Geometry check sheet. Reference: the model listing, model coordinates, mm. A direction names the side the tool comes from. Give positions to 0.01 mm unless a question says otherwise; leave off trailing zeros. Order: outer loops, then holes, each group sorted by start corner. A loop starts at its lowest first (then second) coordinate and runs counter-clockwise, first axis right, second up. Notation, with made-up numbers: M 17.5,62.5 L 47.5,62.5 A17 ccw 47.5,79.5 Z; hole C 5,65 d2. An arc over 180 degrees is marked long. Answer as CSV lines item,"result".
from build123d import *

# Parameters (mm, degrees)
SKETCH1_R           = 6
BOSS_EXTRUDE1_DEPTH = 10
CUT_EXTRUDE1_REACH  = 34.013
CUT_EXTRUDE2_START  = -12.127591
CUT_EXTRUDE2_DEPTH  = 8.847142
BOSS_EXTRUDE7_DEPTH = 5
SKETCH3_R           = 1.25
CUT_EXTRUDE3_DEPTH  = 5
SKETCH3_2_R         = 1.25
CUT_EXTRUDE4_DEPTH  = 11.819305932


with BuildPart() as part:
    # Sketch1 → Boss-Extrude1 (new body)
    with BuildSketch(Plane(origin=(0, 0, 0), x_dir=(0, 0, -1), z_dir=(1, 0, 0))):
        with BuildLine():
            Line((-4.273163423, 7.920863233), (-4.273163423, 20.04845395))
            Line((-4.273163423, 20.04845395), (6, 20.04845395))
            Line((6, 20.04845395), (6, 17.649323049))
            Line((6, 17.649323049), (4.273163423, 17.649323049))
            Line((4.273163423, 17.649323049), (4.273163423, 16.76800454))
            Line((4.273163423, 16.76800454), (5.136581711, 16.76800454))
            Line((5.136581711, 16.76800454), (5.136581711, 15.879894787))
            Line((5.136581711, 15.879894787), (4.273163423, 15.879894787))
            Line((4.273163423, 15.879894787), (4.273163423, 14.998576279))
            Line((4.273163423, 14.998576279), (5.136581711, 14.998576279))
            Line((5.136581711, 14.998576279), (5.136581711, 14.110466526))
            Line((5.136581711, 14.110466526), (4.273163423, 14.110466526))
            Line((4.273163423, 14.110466526), (4.273163423, 13.229148017))
            Line((4.273163423, 13.229148017), (5.136581711, 13.229148017))
            Line((5.136581711, 13.229148017), (5.136581711, 12.341038265))
            Line((5.136581711, 12.341038265), (4.273163423, 12.341038265))
            Line((4.273163423, 12.341038265), (4.273163423, 11.459719756))
            Line((4.273163423, 11.459719756), (5.136581711, 11.459719756))
            Line((5.136581711, 11.459719756), (5.136581711, 10.571610003))
            Line((5.136581711, 10.571610003), (4.273163423, 10.571610003))
            Line((4.273163423, 10.571610003), (4.273163423, 9.690291495))
            Line((4.273163423, 9.690291495), (5.136581711, 9.690291495))
            Line((5.136581711, 9.690291495), (5.136581711, 8.802181742))
            Line((5.136581711, 8.802181742), (4.273163423, 8.802181742))
            Line((4.273163423, 8.802181742), (4.273163423, 7.920863233))
            ThreePointArc((4.273163423, 7.920863233), (0, -9), (-4.273163423, 7.920863233))
        make_face()
        Circle(SKETCH1_R, mode=Mode.SUBTRACT)
    extrude(amount=BOSS_EXTRUDE1_DEPTH)

    # Cut-Extrude1: up to this face of the body (flat: up to its plane)
    cut_extrude1_end = Plane(part.part.faces().sort_by_distance((5, 16.76800454, -4.704872567))[0])
    # Sketch2 → Cut-Extrude1 (cut, up to the picked face)
    with BuildSketch(Plane(origin=(0, 20.04845395, 0), x_dir=(1, 0, 0), z_dir=(0, 1, 0)), mode=Mode.PRIVATE) as cut_extrude1_sk1:
        Polygon((10, 6), (5, 6), (10, 1), align=None)
    cut_extrude1_tool1 = split(extrude(cut_extrude1_sk1.sketch, amount=-CUT_EXTRUDE1_REACH, mode=Mode.PRIVATE), bisect_by=cut_extrude1_end, keep=Keep.BOTH, mode=Mode.PRIVATE)
    # Sketch2 → Cut-Extrude1 (cut, up to the picked face)
    with BuildSketch(Plane(origin=(0, 20.04845395, 0), x_dir=(1, 0, 0), z_dir=(0, 1, 0)), mode=Mode.PRIVATE) as cut_extrude1_sk2:
        Polygon((10, -4.273163423), (10, 0.726836577), (5, -4.273163423), align=None)
    cut_extrude1_tool2 = split(extrude(cut_extrude1_sk2.sketch, amount=-CUT_EXTRUDE1_REACH, mode=Mode.PRIVATE), bisect_by=cut_extrude1_end, keep=Keep.BOTH, mode=Mode.PRIVATE)
    add(cut_extrude1_tool1.solids().sort_by(Axis((8.333333, 20.048454, -4.333333), (0, -1, 0)))[0], mode=Mode.SUBTRACT)
    add(cut_extrude1_tool2.solids().sort_by(Axis((8.333333, 20.048454, 2.606497), (0, -1, 0)))[0], mode=Mode.SUBTRACT)

    # Sketch2<5> → Cut-Extrude2 (cut)
    with BuildSketch(Plane(origin=(0, 20.04845395, 0), x_dir=(1, 0, 0), z_dir=(0, 1, 0)).offset(CUT_EXTRUDE2_START)):
        Polygon((10, -4.273163423), (10, 0.726836577), (5, -4.273163423), align=None)
    extrude(amount=CUT_EXTRUDE2_DEPTH, mode=Mode.SUBTRACT)

    # Sketch2<6> → Boss-Extrude7 (add)
    with BuildSketch(Plane(origin=(0, 20.04845395, 0), x_dir=(1, 0, 0), z_dir=(0, 1, 0))):
        with BuildLine():
            Line((2.586901632, 2.936824491), (2.586901632, -1.209987914))
            ThreePointArc((2.586901632, -1.209987914), (5, -2.400051514), (4.475236793, 0.238872259))
            Line((4.475236793, 0.238872259), (4.475236793, 1.487964318))
            ThreePointArc((4.475236793, 1.487964318), (5, 4.126888091), (2.586901632, 2.936824491))
        make_face()
    extrude(amount=BOSS_EXTRUDE7_DEPTH)

    # Sketch3 → Cut-Extrude3 (cut)
    with BuildSketch(Plane(origin=(0, 25.04845395, 0), x_dir=(1, 0, 0), z_dir=(0, 1, 0))):
        with Locations(Location((4.086901632, 2.936824491, 0), (0, 0, 270))):
            Circle(SKETCH3_R)
        with Locations(Location((4.086901632, -1.209987914, 0), (0, 0, 270))):
            Circle(SKETCH3_R)
    extrude(amount=-CUT_EXTRUDE3_DEPTH, mode=Mode.SUBTRACT)

    # Sketch3<2> → Cut-Extrude4 (cut)
    with BuildSketch(Plane(origin=(0, 25.04845395, 0), x_dir=(1, 0, 0), z_dir=(0, 1, 0))):
        with Locations(Location((4.086901632, 2.936824491, 0), (0, 0, 270))):
            Circle(SKETCH3_2_R)
        with Locations(Location((4.086901632, -1.209987914, 0), (0, 0, 270))):
            Circle(SKETCH3_2_R)
    extrude(amount=-CUT_EXTRUDE4_DEPTH, mode=Mode.SUBTRACT)


solid = part.part
(1) Section check B-B on y = 0. Enter the section's corners in (x, z), then the cut area to 3 significant figures.
The answers:
outline,"M 0,-9 L 10,-9 L 10,-6 L 0,-6 Z; M 0,6 L 10,6 L 10,9 L 0,9 Z"
area,"60.0 mm2"
(2) Tool access check on faces 1 (the face through (5.037, 22.513, -4.098)), 2 (the face through (2, 14, 4.273)), 3 (the face through (4.9, 11.46, -4.7)). Record the directions out of +Z, -Z, +X, -X, +Y, -Y that give a thin tool (end or side, any length) a straight path to the whole face; none if there is none.
The answers:
face 1,"+Y"
face 2,"+Z, +X, -X, +Y"
face 3,"-Z, +X, -X"
(3) Section check A-A on x = 2.25. Enter the section's corners in (y, z), then the cut area to 3 significant figures.
The answers:
outline,"M 7.92,-4.27 L 8.8,-4.27 L 8.8,-5.14 L 9.69,-5.14 L 9.69,-4.27 L 10.57,-4.27 L 10.57,-5.14 L 11.46,-5.14 L 11.46,-4.27 L 12.34,-4.27 L 12.34,-5.14 L 13.23,-5.14 L 13.23,-4.27 L 14.11,-4.27 L 14.11,-5.14 L 15,-5.14 L 15,-4.27 L 15.88,-4.27 L 15.88,-5.14 L 16.77,-5.14 L 16.77,-4.27 L 17.65,-4.27 L 17.65,-6 L 20.05,-6 L 20.05,4.27 L 7.92,4.27 A9 ccw long Z; hole C 0,0 d12"
area,"247 mm2"
(4) Section check D-D on y = 18.5. Enter the section's corners in (x, z).
The answers:
outline,"M 0,-6 L 5,-6 L 10,-1 L 10,-0.73 L 5,4.27 L 0,4.27 Z; hole C 4.09,-2.94 d2.5; hole C 4.09,1.21 d2.5"
(5) Material ranges on line 1 (Y direction, x = 6.75, z = 0); line 2 (X direction, y = 23, z = -3); line 3 (X direction, y = 21.5, z = -0.5), recorded low to high.
The answers:
line 1,"y = -9 to -6, 6 to 20.05"
line 2,"x = 2.59 to 2.84, 5.34 to 5.59"
line 3,"x = 2.59 to 4.48"
(6) Section check C-C on z = -2.25. Enter the section's corners in (x, y).
The answers:
outline,"M 0,-8.71 L 10,-8.71 L 10,-5.56 L 0,-5.56 Z; M 0,5.56 L 10,5.56 L 10,16.77 L 8.75,16.77 L 8.75,20.05 L 5.42,20.05 L 5.42,25.05 L 5.13,25.05 L 5.13,13.23 L 3.04,13.23 L 3.04,25.05 L 2.59,25.05 L 2.59,20.05 L 0,20.05 Z"
(7) Draft check along Z on faces 4 (the face through (3, 17, -4.273)), 5 (the face through (4.9, 12.341, -4.7)), 6 (the face through (4.475, 23, -1)). Enter one of: +Z half, -Z half, draft (parallel to the pull), parting line (faces both ways), or undercut.
The answers:
face 4,"-Z half"
face 5,"draft"
face 6,"undercut"
(8) Gauge pin test, flat ends, axial feed: P1, Ø3, axis at x = 5.5, z = 5, coming from the +Y side; P2, Ø4, axis at x = 1.5, y = 12, coming from the +Z side; P3, Ø0.7, axis at x = 4.5, y = 14.5, coming from the -Z side. Record the tip position at first contact, or that the pin passes through.
The answers:
P1,"stops at y = 20.05"
P2,"stops at z = 4.27"
P3,"stops at z = -5.14"
